Input: part model. Units: mm. Frame: model coordinates. A direction names the side the tool comes from. Round coordinates to 2 decimals unless told otherwise and drop trailing zeros. Write each loop counter-clockwise with the first axis right and the second up, starting at its lowest first coordinate (ties: lowest second). Pieces come first, ordered by that corner, then holes. Notation, with made-up numbers: (59.5, 85.5) -> (98.5, 85.5) arc R13 ccw to (98.5, 108.5) -> close; hole circle Ø6 at (85.5, 41.5). An arc over 180 degrees is marked (long way). Write item = value, one per line.
```python
from build123d import *


with BuildPart() as part:
    # Sketch1 → Revolve1 (revolve)
    with BuildSketch(Plane.XY, mode=Mode.PRIVATE) as revolve1_sk:
        with BuildLine():
            Line((70, 0), (70, 20))
            Line((70, 20), (57, 20))
            ThreePointArc((57, 20), (51.745388578, 21.967665559), (49.075606637, 26.902735298))
            Line((49.075606637, 26.902735298), (33, 143))
            Line((33, 143), (35, 145))
            Line((35, 145), (35, 185))
            Line((35, 185), (25, 185))
            Line((25, 185), (25, 127.867048884))
            Line((25, 127.867048884), (42.289929827, 3))
            Line((42.289929827, 3), (48, 3))
            ThreePointArc((48, 3), (49.414213562, 2.414213562), (50, 1))
            Line((50, 1), (50, 0))
            Line((50, 0), (70, 0))
        make_face()
    revolve(revolve1_sk.sketch.rotate(Axis((0, 99.490022173, 0), (0, -1, 0)), 90), axis=Axis((0, 99.490022173, 0), (0, -1, 0)))


solid = part.part
```
1) Access query for faces 1 (the face through (-0.3, 20, -57.4)), 2 (the face through (-9.95, 143.13, 31.6)), 3 (the face through (42.44, 3, 0.22)). Directions: +Z, -Z, +X, -X, +Y, -Y. A direction counts if a zero-diameter tool reaches every point of the face in a straight line with its end or side. Return the directions, or none.
Solutions:
face_1 = +Y
face_2 = none
face_3 = -Y
2) Cut plane C-C (y = 107.5). Return the cut outline in (x, z).
Solutions:
outline = circle Ø75.83 at (0, 0); hole circle Ø55.64 at (0, 0)
3) Line query: L1, parallel to X at y = 155, z = 0; L2, parallel to X at y = 0.3, z = 0; L3, parallel to Y at x = 52.5, z = -20.5. Output: solid intervals per line, ascending. Write a range as from..to.
Solutions:
L1 = -35..-25, 25..35
L2 = -70..-50, 50..70
L3 = 0..20.03
4) Cut plane D-D (y = 57.5). Return the cut outline in (x, z), and give its area (3 significant figures).
Solutions:
outline = circle Ø89.68 at (0, 0); hole circle Ø69.49 at (0, 0)
area = 2,520 mm^2
5) Draft query along X for faces 4 (the face through (34.168, 165.28, -7.587)), 5 (the face through (-28.472, 64.559, 18.152)), 6 (the face through (-17, 0, 48)). Return one class per face: +X half, -X half, draft (parallel to the pull), parting line (faces both ways), or undercut.
Solutions:
face_4 = parting line
face_5 = undercut
face_6 = draft
6) Cut plane B-B (z = 0). Return the cut outline in (x, y).
Solutions:
outline = (-70, 0) -> (-50, 0) -> (-50, 1) arc R2 cw to (-48, 3) -> (-42.29, 3) -> (-25, 127.87) -> (-25, 185) -> (-35, 185) -> (-35, 145) -> (-33, 143) -> (-49.08, 26.9) arc R8 cw to (-57, 20) -> (-70, 20) -> close; (25, 127.87) -> (42.29, 3) -> (48, 3) arc R2 cw to (50, 1) -> (50, 0) -> (70, 0) -> (70, 20) -> (57, 20) arc R8 cw to (49.08, 26.9) -> (33, 143) -> (35, 145) -> (35, 185) -> (25, 185) -> close
7) First-contact query: P1, Ø5, axis at x = 15.5, y = 67.5, coming from the -Z side; P2, Ø3, axis at y = 24, z = 42, coming from the +X side; P3, Ø10, axis at y = 100.5, z = -24.5, coming from the -X side. Flat tips, straight axial feed; report the tip coordinate or a pass-through.
Solutions:
P1 = -41.54
P2 = 30.08
P3 = -33.75
8) Cut plane A-A (x = 0). Return the cut outline in (y, z), and give its area (3 significant figures).
Solutions:
outline = (0, -70) -> (20, -70) -> (20, -57) arc R8 cw to (26.9, -49.08) -> (143, -33) -> (145, -35) -> (185, -35) -> (185, -25) -> (127.87, -25) -> (3, -42.29) -> (3, -48) arc R2 cw to (1, -50) -> (0, -50) -> close; (0, 50) -> (1, 50) arc R2 cw to (3, 48) -> (3, 42.29) -> (127.87, 25) -> (185, 25) -> (185, 35) -> (145, 35) -> (143, 33) -> (26.9, 49.08) arc R8 cw to (20, 57) -> (20, 70) -> (0, 70) -> close
area = 4,410 mm^2
